Autodesk Inventor part; units mm, degrees
ref_plane "YZ Plane" through (0, 0, 0) normal (1, 0, 0) x (0, 1, 0)
ref_plane "XZ Plane" through (0, 0, 0) normal (0, 1, 0) x (-1, 0, 0)
ref_plane "XY Plane" through (0, 0, 0) normal (0, 0, 1) x (1, 0, 0)
sketch "Sketch1" plane through (0, 0, 0) normal (0, 1, 0) x (-1, 0, 0)
  arc A0 (5.6966, -10.4681) -> (3.0156, -10.4681) centre (4.3561, -12.7) ccw
  line L0 (17.0561, -25.4) -> (-8.3439, -25.4)
  line L1 (-8.3439, -25.4) -> (-8.3439, 0)
  line L2 (17.0561, 0) -> (17.0561, -25.4)
  line L3 (17.0561, -25.4) -> (-8.3439, 0) construction
  line L4 (-8.3439, -25.4) -> (17.0561, 0) construction
  line L5 (-14.7304, 17.477) -> (-14.7304, -47.796)
  line L6 (-14.7304, -47.796) -> (26.0883, -47.796)
  line L7 (26.0883, -47.796) -> (26.0883, 17.477)
  line L8 (-1.3293, 0) -> (-1.3293, 17.477)
  line L9 (6.9778, 17.477) -> (6.9778, 0)
  line L10 (-8.3439, 0) -> (-1.3293, 0)
  line L11 (6.9778, 0) -> (17.0561, 0)
  line L12 (26.0883, 17.477) -> (6.9778, 17.477)
  line L13 (-1.3293, 17.477) -> (-14.7304, 17.477)
  point P0 (0, 0)
  dimension "d0" = 25.4
  dimension "d1" = 25.4
extrude "Extrusion1" add sketch "Sketch1" along normal mid plane 38.1
sketch "Sketch2" plane through (14.7304, -19.05, -47.796) normal (1, 0, 0) x (0, 0, -1)
  arc A0 (-22.6007, 24.7617) -> (-22.396, 13.1445) centre (-16.9992, 19.05) ccw
  circle A1 centre (-16.9992, 19.05) radius 8
  circle A2 centre (-16.9992, 19.05) radius 8.0635
  point P0 (-47.796, 19.05)
  dimension "d4" = 0.0635
extrude "Extrusion2" cut sketch "Sketch2" against normal through all contours A1 A0 | A2
fillet "Fillet1" radius 12.7 2 edges at (-5.6789, -19.05, -47.796) (-5.6789, 19.05, -47.796)
fillet "Fillet2" radius 3.175 4 edges at (8.0299, 19.05, 17.477) (-16.533, 19.05, 17.477) (-16.533, -19.05, 17.477) (8.0299, -19.05, 17.477)
sketch "Sketch3" plane through (14.7304, -6.35, -47.796) normal (1, 0, 0) x (0, 0, -1)
  circle A0 centre (-16.9992, 6.35) radius 8.0635
  arc A1 (-65.2731, -9.525) -> (-62.0981, -12.7) centre (-62.0981, -9.525) ccw
  line L0 (-12.7, -12.7) -> (-62.0981, -12.7)
  arc A2 (-12.7, -12.7) -> (0, 0) centre (-12.7, 0) ccw
  line L1 (0, 0) -> (0, 12.7)
  arc A3 (0, 12.7) -> (-12.7, 25.4) centre (-12.7, 12.7) ccw
  line L2 (-62.0981, 25.4) -> (-12.7, 25.4)
  arc A4 (-62.0981, 25.4) -> (-65.2731, 22.225) centre (-62.0981, 22.225) ccw
  line L3 (-65.2731, -9.525) -> (-65.2731, 22.225)
  line L4 (-48.1725, 17.0318) -> (-55.7015, 17.0318) construction
  line L5 (-55.7015, 17.0318) -> (-55.7015, -4.3318) construction
  line L6 (-55.7015, -4.3318) -> (-48.1725, -4.3318) construction
  line L7 (-48.1725, -4.3318) -> (-48.1725, 17.0318) construction
  line L8 (-48.1725, 17.0318) -> (-55.7015, -4.3318) construction
  line L9 (-55.7015, 17.0318) -> (-48.1725, -4.3318) construction
  circle A5 centre (-55.7015, 17.0318) radius 2.625
  circle A6 centre (-55.7015, -4.3318) radius 2.625
  point P0 (-47.796, 6.35)
  point P1 (-51.937, 6.35)
  dimension "d9" = 5.25
  dimension "d10" = 5.25
extrude "Extrusion3" cut sketch "Sketch3" against normal through all contours A5 | A6
sketch "Sketch4" plane through (-26.0883, -6.35, -47.796) normal (-1, 0, 0) x (0, 0, 1)
  circle A0 centre (55.7015, 17.0318) radius 2.625
  circle A1 centre (55.7015, -4.3318) radius 2.625
  circle A2 centre (16.9992, 6.35) radius 8.0635
  arc A3 (62.0981, -12.7) -> (65.2731, -9.525) centre (62.0981, -9.525) ccw
  line L0 (65.2731, -9.525) -> (65.2731, 22.225)
  arc A4 (65.2731, 22.225) -> (62.0981, 25.4) centre (62.0981, 22.225) ccw
  line L1 (12.7, 25.4) -> (62.0981, 25.4)
  arc A5 (12.7, 25.4) -> (0, 12.7) centre (12.7, 12.7) ccw
  line L2 (0, 0) -> (0, 12.7)
  arc A6 (0, 0) -> (12.7, -12.7) centre (12.7, 0) ccw
  line L3 (62.0981, -12.7) -> (12.7, -12.7)
  line L4 (60.3203, 17.0318) -> (58.0109, 13.0318)
  line L5 (58.0109, 13.0318) -> (53.3921, 13.0318)
  line L6 (53.3921, 13.0318) -> (51.0827, 17.0318)
  line L7 (51.0827, 17.0318) -> (53.3921, 21.0318)
  line L8 (53.3921, 21.0318) -> (58.0109, 21.0318)
  line L9 (58.0109, 21.0318) -> (60.3203, 17.0318)
  line L10 (60.3203, -4.3318) -> (58.0109, -8.3318)
  line L11 (58.0109, -8.3318) -> (53.3921, -8.3318)
  line L12 (53.3921, -8.3318) -> (51.0827, -4.3318)
  line L13 (51.0827, -4.3318) -> (53.3921, -0.3318)
  line L14 (53.3921, -0.3318) -> (58.0109, -0.3318)
  line L15 (58.0109, -0.3318) -> (60.3203, -4.3318)
  point P0 (47.796, 6.35)
  dimension "d13" = 8
  dimension "d14" = 8
extrude "Extrusion4" cut sketch "Sketch4" against normal blind 12.7 contours L4 L5 L6 L7 L8 L9 | L10 L11 L12 L13 L14 L15
sketch "Sketch5" plane through (14.7304, -6.35, -47.796) normal (1, 0, 0) x (0, 0, -1)
  circle A0 centre (-55.7015, 17.0318) radius 2.625
  circle A1 centre (-55.7015, -4.3318) radius 2.625
  circle A2 centre (-16.9992, 6.35) radius 8.0635
  arc A3 (-65.2731, -9.525) -> (-62.0981, -12.7) centre (-62.0981, -9.525) ccw
  line L0 (-12.7, -12.7) -> (-62.0981, -12.7)
  arc A4 (-12.7, -12.7) -> (0, 0) centre (-12.7, 0) ccw
  line L1 (0, 0) -> (0, 12.7)
  arc A5 (0, 12.7) -> (-12.7, 25.4) centre (-12.7, 12.7) ccw
  line L2 (-62.0981, 25.4) -> (-12.7, 25.4)
  arc A6 (-62.0981, 25.4) -> (-65.2731, 22.225) centre (-62.0981, 22.225) ccw
  line L3 (-65.2731, -9.525) -> (-65.2731, 22.225)
  circle A7 centre (-55.7015, -4.3318) radius 2.625
  circle A8 centre (-55.7015, -4.3318) radius 5
  circle A9 centre (-55.7015, 17.0318) radius 5
  point P0 (-47.796, 6.35)
  dimension "d17" = 10
  dimension "d18" = 10
extrude "Extrusion5" cut sketch "Sketch5" against normal blind 6.35 contours A8 | A9
properties part number "3d printed motor shaft block for base v1"
Read the model definition and answer for the solid it produces. Units are mm, in the model's axes. A direction names the side the tool comes from. Give positions to 0.01 mm unless a question says otherwise; leave off trailing zeros. Loops run counter-clockwise (first coordinate to the right, second up) from the corner with the lowest first, then second, coordinate; pieces in that order, holes last.
Item 1: Each of these flat-tipped pins is pushed along its axis until it touches: pin 1 Ø6 at (y, z) = (-10.68, 7.91) entering from -X; pin 2 Ø3 at (y, z) = (13, 9) entering from +X; pin 3 Ø3 at (y, z) = (-10.68, 7.91) entering from -X (1 decimal). Where does it stop, or does it pass through?
Item 2: The part is cut by section C-C (z = -28). Write down the section's boundary in (x, y), and give its area (3 significant figures).
Item 3: The part is cut by section A-A (x = -8.5). Give the number of separate pieces and of enclosed holes in the cut face, and give its area (3 significant figures).
Item 4: Find the intervals of material crossed by line 1 along Y through (x, z) = (-22, 8.5); line 2 along X through (y, z) = (-7, 9.5); line 3 along Z through (x, y) = (3, 0), in increasing order.
Item 5: The mould has two halves that part along Z. Classify faces 6 (the flat face through (-5, 0, -47.796)), 7 (the cylindrical face through (4.9, -13.01, 6.69)), 8 (the cylindrical face through (8.124, 18.145, 16.522)): released by +Z, released by -Z, zero draft, split by the parting line, or undercut.
Item 6: For faces 1 (the cylindrical face through (-10.1, 12.9, 6.5)), 2 (the flat face through (-6.978, 0, 9)), 3 (the flat face through (8.344, 0, -13)), 4 (the cylindrical face through (-16.399, 18.145, 16.522)), 5 (the flat face through (-20, -6.682, 8)), determine the directions among +Z, -Z, +X, -X, +Y, -Y from which every point of the face is accessible in a straight line to the end or side of a thin tool.
Item 7: The part is cut by section B-B (y = 0). Write down the section's boundary in (x, z), and give its area (3 significant figures).
Taken from the geometry:
1. pin 1: stops at x = -13.39
1. pin 2: stops at x = 8.38
1. pin 3: passes through
2. outline: (-26.09, -19.05) - (14.73, -19.05) - (14.73, -7.56) - (-26.09, -7.56) - close; (-26.09, 7.56) - (14.73, 7.56) - (14.73, 19.05) - (-26.09, 19.05) - close
2. area: 938 mm2
3. separate pieces: 2
3. enclosed holes: 2
3. area: 1,220 mm2
4. line 1: y = -19.05 to -14.68, -6.68 to 6.68, 14.68 to 19.05
4. line 2: x = -13.39 to -6.98, 1.33 to 8.38
4. line 3: z = -47.8 to -38.86, 0 to 17.48
5. face 6: released by -Z
5. face 7: undercut
5. face 8: released by +Z
6. face 1: +X, -X
6. face 2: +Z, +Y, -Y
6. face 3: +Y, -Y
6. face 4: +Z, +X, -X, +Y
6. face 5: -X
7. outline: (-26.09, -47.8) - (14.73, -47.8) - (14.73, -38.86) - (-26.09, -38.86) - close; (-26.09, -22.73) - (-17.06, -22.73) - (-17.06, 0) - (-6.98, 0) - (-6.98, 17.48) - (-26.09, 17.48) - close; (1.33, 0) - (8.34, 0) - (8.34, -22.73) - (14.73, -22.73) - (14.73, 17.48) - (1.33, 17.48) - close
7. area: 1,280 mm2
